from build123d import *

# Parameters (mm, degrees)
PAD_DEPTH          = 8
SKETCH001_W        = 24.2
SKETCH001_H        = 8.6
POCKET_DEPTH       = 433.263242
POLARPATTERN_COUNT = 3


with BuildPart() as part:
    # Sketch → Pad (new body)
    with BuildSketch(Plane.XY):
        with BuildLine():
            Line((51.5303, 115.351058), (57.5303, 115.351058))
            Line((57.5303, 115.351058), (57.5303, 17.037153))
            ThreePointArc((-15.362291, 58), (-29.394284, -52.306558), (57.5303, 17.037153))
            Line((43.5303, 67.351058), (-15.362291, 58))
            Line((51.5303, 67.351058), (43.5303, 67.351058))
            Line((51.5303, 75.351058), (51.5303, 67.351058))
            Line((43.5303, 75.351058), (51.5303, 75.351058))
            Line((43.5303, 83.351058), (43.5303, 75.351058))
            Line((51.5303, 83.351058), (43.5303, 83.351058))
            Line((51.5303, 91.351058), (51.5303, 83.351058))
            Line((43.5303, 91.351058), (51.5303, 91.351058))
            Line((43.5303, 99.351058), (43.5303, 91.351058))
            Line((51.5303, 99.351058), (43.5303, 99.351058))
            Line((51.5303, 107.351058), (51.5303, 99.351058))
            Line((43.5303, 107.351058), (51.5303, 107.351058))
            Line((43.5303, 115.351058), (43.5303, 107.351058))
            Line((51.5303, 115.351058), (43.5303, 115.351058))
        make_face()
    extrude(amount=PAD_DEPTH)

    # Sketch001 → Pocket (cut, through all)
    with BuildSketch(Plane.XY.offset(8)):
        with Locations((0, -40)):
            Rectangle(SKETCH001_W, SKETCH001_H)
    pocket = extrude(amount=-POCKET_DEPTH, mode=Mode.SUBTRACT)

    # PolarPattern: Pocket ×3 about axis
    polarpattern_axis = Axis((0, 0, 8), (0, 0, 1))
    for i in range(1, POLARPATTERN_COUNT):
        add(pocket.rotate(polarpattern_axis, i * 360 / POLARPATTERN_COUNT), mode=Mode.SUBTRACT)


solid = part.part
Work out the finished part from the listing and answer in its coordinate system (mm). A direction names the side the tool comes from. Round coordinates to 2 decimals unless told otherwise and drop trailing zeros. Write each loop counter-clockwise with the first axis right and the second up, starting at its lowest first coordinate (ties: lowest second). Pieces come first, ordered by that corner, then holes.
1) A tool of negligible diameter and unlimited length cuts with its end or side. For faces 3 (the flat face through (1, 9, 8)), 4 (the flat face through (-40.74, 9.55, 4.06)), 5 (the flat face through (1, 9, 0)), 6 (the flat face through (43.53, 111, 4)), 7 (the flat face through (47, 91.351, 4)), from which of +Z, -Z, +X, -X, +Y, -Y can it reach the whole face along a straight path? Write none if from no direction.
2) A cutting plane is placed at C-C (y = 105). Give the vertices of the cut face in (x, z), plus the area to 3 significant figures.
3) A cutting plane is placed at D-D (y = 44.5). Give the vertices of the cut face in (x, z), plus the area to 3 significant figures.
4) Straight lines are drawn through the part: line 1 (X direction, y = 27, z = 6.5); line 2 (X direction, y = 22.5, z = 1.75); line 3 (Y direction, x = 3, z = 3). For each, find the intervals that lie inside material, in ascending order.
5) The mould has two halves that part along Y. Classify faces 1 (the flat face through (43.53, 95, 4)), 2 (the flat face through (47, 75.351, 4)): pulls with the +Y half, pulls with the -Y half, needs draft (parallel to the pull), parting line crosses it, or undercut.
6) Given pin 1 Ø2.5 at (x, z) = (-4, 6) entering from +Y; pin 2 Ø2.5 at (y, z) = (95, 3.5) entering from -X; pin 3 Ø4 at (y, z) = (70.5, 3.5) entering from -X, each flat-ended and moving along its own axis, determine where each tip first touches the part or whether it passes through.
7) A cutting plane is placed at B-B (x = 0). Give the vertices of the cut face in (y, z), plus the area to 3 significant figures.
8) A cutting plane is placed at A-A (z = 5.75). Give the vertices of the cut face in (x, y), plus the area to 3 significant figures.
Completed:
1. face 3: +Z, +X, -X, +Y, -Y
1. face 4: +Z, -Z
1. face 5: -Z, +X, -X, +Y, -Y
1. face 6: +Z, -Z, -X, +Y
1. face 7: +Z, -Z, -X
2. outline: (51.53, 0) - (57.53, 0) - (57.53, 8) - (51.53, 8) - close
2. area: 48.0 mm2
3. outline: (-40.25, 0) - (57.53, 0) - (57.53, 8) - (-40.25, 8) - close
3. area: 782 mm2
4. line 1: x = -53.58 to -35.56, -25.63 to 25.63, 35.56 to 57.53
4. line 2: x = -55.62 to -38.16, -28.23 to 28.23, 38.16 to 57.53
4. line 3: y = -59.92 to -44.3, -35.7 to 60.92
5. face 1: needs draft
5. face 2: undercut
6. pin 1: stops at y = 60
6. pin 2: stops at x = 43.53
6. pin 3: stops at x = 51.53
7. outline: (-60, 0) - (-44.3, 0) - (-44.3, 8) - (-60, 8) - close; (-35.7, 0) - (60.44, 0) - (60.44, 8) - (-35.7, 8) - close
7. area: 895 mm2
8. outline: (-15.36, 58) arc R60 ccw (long way) to (57.53, 17.04) - (57.53, 115.35) - (43.53, 115.35) - (43.53, 107.35) - (51.53, 107.35) - (51.53, 99.35) - (43.53, 99.35) - (43.53, 91.35) - (51.53, 91.35) - (51.53, 83.35) - (43.53, 83.35) - (43.53, 75.35) - (51.53, 75.35) - (51.53, 67.35) - (43.53, 67.35) - close; hole (-44.41, 11.67) - (-36.97, 7.37) - (-24.87, 28.33) - (-32.31, 32.63) - close; hole (-12.1, -44.3) - (12.1, -44.3) - (12.1, -35.7) - (-12.1, -35.7) - close; hole (24.87, 28.33) - (36.97, 7.37) - (44.41, 11.67) - (32.31, 32.63) - close
8. area: 12,100 mm2
